from build123d import *

# Parameters (mm, degrees)
BOSS_EXTRUDE1_DEPTH  = 2032
LPATTERN1_COUNT      = 6
LPATTERN1_PITCH      = 130.66776
LPATTERN1_COUNT_DIR2 = 7
LPATTERN1_PITCH_DIR2 = 130.66776
CUT_EXTRUDE1_DEPTH   = 2032


with BuildPart() as part:
    # Sketch1 → Boss-Extrude1 (new body)
    with BuildSketch(Plane.XY):
        Polygon((0, 0), (12.7, 0), (52.634727814, 762), (78.034727814, 762), (117.969455627, 0), (130.669455627, 0), (130.669455627, -127), (0, -127), align=None)
    boss_extrude1 = extrude(amount=-BOSS_EXTRUDE1_DEPTH)

    # LPattern1: Boss-Extrude1 6 × 7
    with Locations(*[Vector(-1, 0, 0) * (i * LPATTERN1_PITCH) + Vector(1, 0, 0) * (j * LPATTERN1_PITCH_DIR2) for i in range(LPATTERN1_COUNT) for j in range(LPATTERN1_COUNT_DIR2) if (i, j) != (0, 0)]):
        add(boss_extrude1)

    # Sketch2 → Cut-Extrude1 (cut)
    with BuildSketch(Plane.XY):
        Polygon((-640.6388, 0), (-647.294587969, -127), (-653.3388, -127), (-653.3388, 0), align=None)
        Polygon((901.976015627, 0), (908.631803596, -127), (914.676015627, -127), (914.676015627, 0), align=None)
    extrude(amount=-CUT_EXTRUDE1_DEPTH, mode=Mode.SUBTRACT)


solid = part.part
Input: part model. Units: mm. Frame: model coordinates. A direction names the side the tool comes from. Give positions to 0.01 mm unless a question says otherwise; leave off trailing zeros. Use one line per item in the form item = value. Start each with the question number.
1) Section query A-A on y = 165. Count the separate pieces of the cut face and the enclosed holes in it, then the cut area to 3 significant figures.
2) Set-up query: faces 1 (the flat face through (314, 225, 0)), 2 (the flat face through (816.394, 375.666, -1001.776)). Return all of +Z, -Z, +X, -X, +Y, -Y with unobstructed straight access to the full face (end or side cutting, diameter ignored); none if empty.
3) Pin query (flat end, axial travel): pin 1 (20.5 mm diameter, centred on x = 132.5, z = -622, fed in from +Y); pin 2 (1.5 mm diameter, centred on y = 466, z = -335, fed in from +X); pin 3 (12 mm diameter, centred on y = 626.5, z = -1494, fed in from +X). Return the tip coordinate at first contact, or that it passes through.
4) Draft query along X for faces 3 (the flat face through (555.06, 375.67, -1001.78)), 4 (the flat face through (142, -127, -1002)). Return one class per face: pulls with the +X half, pulls with the -X half, needs draft (parallel to the pull), parting line crosses it, or undercut.
5) Ray query, probe 1 along Y at (x, z) = (-379.5, -644.5); probe 2 along X at (y, z) = (-3.5, -1749.5). Return the intervals inside material, ascending. Write a range as from..to.
Outcome:
q1.separate_pieces = 12
q1.enclosed_holes = 0
q1.area = 2,150,000 mm^2
q2.face_1 = +Z, +X, -X, +Y, -Y
q2.face_2 = +Z, -Z, +Y
q3.pin_1 = 0
q3.pin_2 = 877.59
q3.pin_3 = 869.46
q4.face_3 = undercut
q4.face_4 = needs draft
q5.probe_1 = -127..0
q5.probe_2 = -640.82..902.16
